The drawing under review shows one solid part. Ordinate dimensions are in mm from its lowest x, y, z. Give positions to 0.01 mm unless a question says otherwise; leave off trailing zeros. Order: outer loops, then holes, each group sorted by start corner. A loop starts at its lowest first (then second) coordinate and runs counter-clockwise, first axis right, second up. Notation, with made-up numbers: (4.5, 89.5) -> (50.5, 89.5) arc R31 ccw to (50.5, 125.5) -> close; hole circle Ø9 at (-20.75, 51). An arc over 180 degrees is marked (long way). One line per item, written item: value.
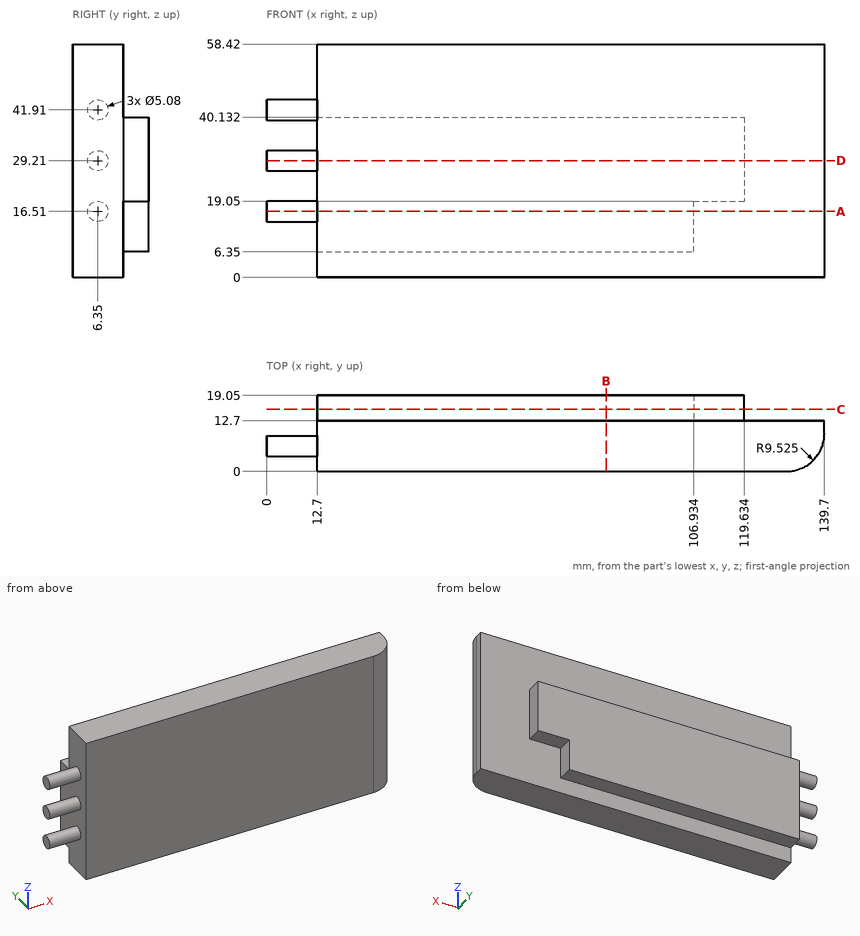
Item 1: Add section D-D on z = 29.21. Give the boundary of the cut face in (x, y) (3 decimals).
Returned:
outline: (0, 3.81) -> (12.7, 3.81) -> (12.7, 0) -> (130.175, 0) arc R9.525 ccw to (139.7, 9.525) -> (139.7, 12.7) -> (119.634, 12.7) -> (119.634, 19.05) -> (12.7, 19.05) -> (12.7, 8.89) -> (0, 8.89) -> close
Item 2: Add section C-C on y = 15.5. Give the boundary of the cut face in (x, z).
Returned:
outline: (12.7, 6.35) -> (106.93, 6.35) -> (106.93, 19.05) -> (119.63, 19.05) -> (119.63, 40.13) -> (12.7, 40.13) -> close
Item 3: To check wall thickness, follow line 1 along Z through (x, y) = (12, 7.25); line 2 along X through (y, z) = (9, 25.5); line 3 along Z through (x, y) = (111, 17.75). State the ranges of each line that lie inside material, in increasing order. Write a range as from..to.
Returned:
line 1: 14.13..18.89, 26.83..31.59, 39.53..44.29
line 2: 12.7..139.69
line 3: 19.05..40.13
Item 4: Add section B-B on x = 85. Give the boundary of the cut face in (y, z).
Returned:
outline: (0, 0) -> (12.7, 0) -> (12.7, 6.35) -> (19.05, 6.35) -> (19.05, 40.13) -> (12.7, 40.13) -> (12.7, 58.42) -> (0, 58.42) -> close
Item 5: Clearance check with flat-ended pins moving along their axes: P1, Ø1.9, axis at y = 17.5, z = 34, coming from the +X side; P2, Ø1.9, axis at x = 63, y = 15, coming from the +Z side; P3, Ø5.5, axis at y = 7, z = 23, coming from the -X side. State where each tip first meets the part, or that it passes through.
Returned:
P1: x = 119.63
P2: z = 40.13
P3: x = 12.7
Item 6: Add section A-A on z = 16.51. Give the boundary of the cut face in (x, y) (3 decimals).
Returned:
outline: (0, 3.81) -> (12.7, 3.81) -> (12.7, 0) -> (130.175, 0) arc R9.525 ccw to (139.7, 9.525) -> (139.7, 12.7) -> (106.934, 12.7) -> (106.934, 19.05) -> (12.7, 19.05) -> (12.7, 8.89) -> (0, 8.89) -> close
